Geometry: final body of the model. Coordinates: model frame, mm. A direction names the side the tool comes from. Give positions to 0.01 mm unless a question says otherwise; leave off trailing zeros. Loops run counter-clockwise (first coordinate to the right, second up) from the corner with the lowest first, then second, coordinate; pieces in that order, holes last. Notation, with made-up numbers: (17, 7) - (28, 7) arc R27 ccw to (28, 39) - close; hole circle Ø2 at (-33, 72.5). An arc over 180 degrees is marked (long way). Use one line per item in the form item = value.
```python
from build123d import *

# Parameters (mm, degrees)
F1_DEPTH = 50.8
F3_DEPTH = 901.7
F4_R     = 31.75
F5_DEPTH = 304.8


with BuildPart() as f1:
    # F0 (on Top) → F1 (new body)
    with BuildSketch(Plane.XY):
        Polygon((25.4, 419.1), (-25.4, 419.1), (-25.4, 25.4), (-419.1, 25.4), (-419.1, -25.4), (-25.4, -25.4), (-25.4, -419.1), (25.4, -419.1), (25.4, -25.4), (419.1, -25.4), (419.1, 25.4), (25.4, 25.4), align=None)
    extrude(amount=F1_DEPTH)

    # F2 (on face) → F3 (join)
    with BuildSketch(Plane.XY.offset(50.8)):
        with BuildLine():
            ThreePointArc((-25.4, 380.15239), (0, 381), (25.4, 380.15239))
            Line((25.4, 380.15239), (25.4, 419.1))
            Line((25.4, 419.1), (-25.4, 419.1))
            Line((-25.4, 419.1), (-25.4, 380.15239))
        make_face()
        with BuildLine():
            ThreePointArc((-380.15239, -25.4), (-381, 0), (-380.15239, 25.4))
            Line((-380.15239, 25.4), (-419.1, 25.4))
            Line((-419.1, 25.4), (-419.1, -25.4))
            Line((-419.1, -25.4), (-380.15239, -25.4))
        make_face()
        with BuildLine():
            Line((25.4, -419.1), (25.4, -380.15239))
            ThreePointArc((25.4, -380.15239), (0, -381), (-25.4, -380.15239))
            Line((-25.4, -380.15239), (-25.4, -419.1))
            Line((-25.4, -419.1), (25.4, -419.1))
        make_face()
        with BuildLine():
            ThreePointArc((380.15239, 25.4), (380.788039, 12.707069), (381, 0))
            ThreePointArc((381, 0), (380.788039, -12.707069), (380.15239, -25.4))
            Line((380.15239, -25.4), (419.1, -25.4))
            Line((419.1, -25.4), (419.1, 25.4))
            Line((419.1, 25.4), (380.15239, 25.4))
        make_face()
    extrude(amount=F3_DEPTH)

    # F4 (on face) → F5 (join)
    with BuildSketch(Plane(origin=(0, 0, 0), x_dir=(1, 0, 0), z_dir=(0, 0, -1))):
        Circle(F4_R)
    extrude(amount=F5_DEPTH)


solid = f1.part
```
(1) Cut plane C-C (z = 24). Return the cut outline in (x, y), plus the area to 3 significant figures.
Solution:
outline = (-419.1, -25.4) - (-25.4, -25.4) - (-25.4, -419.1) - (25.4, -419.1) - (25.4, -25.4) - (419.1, -25.4) - (419.1, 25.4) - (25.4, 25.4) - (25.4, 419.1) - (-25.4, 419.1) - (-25.4, 25.4) - (-419.1, 25.4) - close
area = 82,600 mm2
(2) Cut plane A-A (z = 357.5). Return the cut outline in (x, y).
Solution:
outline = (-419.1, -25.4) - (-380.15, -25.4) arc R381 cw to (-380.15, 25.4) - (-419.1, 25.4) - close; (-25.4, -419.1) - (25.4, -419.1) - (25.4, -380.15) arc R381 cw to (-25.4, -380.15) - close; (-25.4, 380.15) arc R381 cw to (25.4, 380.15) - (25.4, 419.1) - (-25.4, 419.1) - close; (380.15, -25.4) - (419.1, -25.4) - (419.1, 25.4) - (380.15, 25.4) arc R381 cw to (381, 0) arc R381 cw to start
(3) Pin query (flat end, axial travel): P1, Ø4, axis at x = 103.5, y = 20, coming from the +Z side; P2, Ø12, axis at x = 56, y = -10, coming from the -Z side. Return the tip coordinate at first contact, or that it passes through.
Solution:
P1 = 50.8
P2 = 0
(4) Pull-direction query (Y, two-part tool) for faces 1 (the face through (419.1, 0, 470)), 2 (the face through (-2, 2, 50.8)), 3 (the face through (-384, -25.4, 333)); classes: released by +Y, released by -Y, zero draft, split by the parting line, or undercut.
Solution:
face_1 = zero draft
face_2 = undercut
face_3 = released by -Y
(5) Cut plane D-D (y = -117.5). Return the cut outline in (x, z).
Solution:
outline = (-25.4, 0) - (25.4, 0) - (25.4, 50.8) - (-25.4, 50.8) - close
(6) Access query for faces 4 (the face through (-25.4, -382, 298)), 5 (the face through (25.4, -384, 333)), 6 (the face through (384, 25.4, 333)), 7 (the face through (-6.883, 30.995, -150.266)), 8 (the face through (0, -381, 495)). Directions: +Z, -Z, +X, -X, +Y, -Y. A direction counts if a zero-diameter tool reaches every point of the face in a straight line with its end or side. Return the directions, or none.
Solution:
face_4 = +Z, -Z, -X, -Y
face_5 = +Z, -Z, +X, -Y
face_6 = +Z, -Z, +X, +Y
face_7 = -Z
face_8 = +Z
(7) Cut plane B-B (x = 0). Return the cut outline in (y, z).
Solution:
outline = (-419.1, 0) - (-31.75, 0) - (-31.75, -304.8) - (31.75, -304.8) - (31.75, 0) - (419.1, 0) - (419.1, 952.5) - (381, 952.5) - (381, 50.8) - (-381, 50.8) - (-381, 952.5) - (-419.1, 952.5) - close
(8) Material intervals for L1, parallel to X at y = -332.5, z = 36; L2, parallel to Y at x = -24.5, z = 107; L3, parallel to Y at x = -17, z = 799, sorted ascending. Write a range as from..to.
Solution:
L1 = -25.4..25.4
L2 = -419.1..-380.21, 380.21..419.1
L3 = -419.1..-380.62, 380.62..419.1
